```python
from build123d import *

# Parameters (mm, degrees)
BOSS_EXTRUDE1_DEPTH     = 19.05
CUT_EXTRUDE3_DEPTH      = 122.316579658
CUT_EXTRUDE3_DEPTH_BACK = 122.316579658
SKETCH2_R               = 6.35
SKETCH2_R_2             = 16.51


with BuildPart() as part:
    # Sketch1 → Boss-Extrude1 (new body)
    with BuildSketch(Plane.XY):
        Polygon((0, 0), (101.6, 0), (101.6, 44.45), (68.604432116, 63.5), (32.995567884, 63.5), (0, 44.45), align=None)
    extrude(amount=BOSS_EXTRUDE1_DEPTH)

    # Sketch2 → Cut-Extrude3 (cut, two sides: drawn at the far end of the back side and taken through both)
    with BuildSketch(Plane.XY.offset(-CUT_EXTRUDE3_DEPTH_BACK)):
        with Locations(Location((19.05, 19.05, 0), (0, 0, 180))):
            Circle(SKETCH2_R)
        with Locations(Location((82.55, 19.05, 0), (0, 0, 180))):
            Circle(SKETCH2_R)
        with Locations(Location((50.8, 31.75, 0), (0, 0, 180))):
            Circle(SKETCH2_R_2)
    extrude(amount=CUT_EXTRUDE3_DEPTH + CUT_EXTRUDE3_DEPTH_BACK, mode=Mode.SUBTRACT)


solid = part.part
```
Geometry check sheet. Reference: the model listing, model coordinates, mm. Round coordinates to 2 decimals unless told otherwise and drop trailing zeros. Order: outer loops, then holes, each group sorted by start corner. A loop starts at its lowest first (then second) coordinate and runs counter-clockwise, first axis right, second up. Notation, with made-up numbers: (72, 48) - (120, 48) arc R19 ccw to (120, 66) - close; hole circle Ø6 at (-2.75, 57.25). An arc over 180 degrees is marked (long way). Use a Markdown table: item, result. Add a question column.
1) Section check A-A (x = 57). Record the cut outline in (y, z).
2) Section check C-C (y = 19.05). Record the cut outline in (x, z), then the cut area to 3 significant figures.
3) Thickness scan on line 1 along X through (y, z) = (32.5, 10.5); line 2 along Y through (x, z) = (50.8, 6.5); line 3 along X through (y, z) = (35.5, 8). Record the ranges inside material, lowest first.
4) Section check B-B (z = 16.75). Record the cut outline in (x, y).
5) Mould release check, pull along Y, two halves, no side actions. Record for faces 1 (the cylindrical face through (67.294, 31.024, 9.392)), 2 (the flat face through (101.6, 22, 9)), 3 (the flat face through (51, 63.5, 9)): released by +Y, released by -Y, zero draft, split by the parting line, or undercut.
6) Section check D-D (y = 38). Record the cut outline in (x, z), then the cut area to 3 significant figures.
Established:
| question | item | result |
|---|---|---|
| 1 | outline | (0, 0) - (16.45, 0) - (16.45, 19.05) - (0, 19.05) - close; (47.05, 0) - (63.5, 0) - (63.5, 19.05) - (47.05, 19.05) - close |
| 2 | outline | (0, 0) - (12.7, 0) - (12.7, 19.05) - (0, 19.05) - close; (25.4, 0) - (40.25, 0) - (40.25, 19.05) - (25.4, 19.05) - close; (61.35, 0) - (76.2, 0) - (76.2, 19.05) - (61.35, 19.05) - close; (88.9, 0) - (101.6, 0) - (101.6, 19.05) - (88.9, 19.05) - close |
| 2 | area | 1,050 mm2 |
| 3 | line 1 | 0 to 34.31, 67.29 to 101.6 |
| 3 | line 2 | 0 to 15.24, 48.26 to 63.5 |
| 3 | line 3 | 0 to 34.72, 66.88 to 101.6 |
| 4 | outline | (0, 0) - (101.6, 0) - (101.6, 44.45) - (68.6, 63.5) - (33, 63.5) - (0, 44.45) - close; hole circle Ø12.7 at (19.05, 19.05); hole circle Ø33.02 at (50.8, 31.75); hole circle Ø12.7 at (82.55, 19.05) |
| 5 | face 1 | undercut |
| 5 | face 2 | zero draft |
| 5 | face 3 | released by +Y |
| 6 | outline | (0, 0) - (35.52, 0) - (35.52, 19.05) - (0, 19.05) - close; (66.08, 0) - (101.6, 0) - (101.6, 19.05) - (66.08, 19.05) - close |
| 6 | area | 1,350 mm2 |
